Geometry: see drawing. Coordinates: mm, zero at the bounding-box minimum. A direction names the side the tool comes from. Coordinates: 2 decimals unless noted, no trailing zeros. One line per item, written item: value. Start each with the question number.
Item 1: Mould query, pull axis Z, two halves, no side actions, for the marked faces 4, 5, 6 and 7. Classes: released by +Z, released by -Z, zero draft, split by the parting line, or undercut.
Item 2: Pin query (flat end, axial travel): P1, Ø5, axis at x = 30.16, z = 4.76, coming from the -Y side; P2, Ø3, axis at y = 2, z = 3, coming from the -X side; P3, Ø3, axis at x = 31, y = 2, coming from the +Z side (1 decimal); P4, Ø3, axis at y = 1.5, z = 26.5, coming from the +X side (1 decimal). Return the tip coordinate at first contact, or that it passes through.
Item 3: Set-up query: the marked faces 1, 2 and 3. Return all of +Z, -Z, +X, -X, +Y, -Y with unobstructed straight access to the full face (end or side cutting, diameter ignored); none if empty.
Item 4: Ray query, L1, parallel to X at y = 2.5, z = 23 (1 decimal); L2, parallel to Z at x = 17.5, y = 5.75 (1 decimal); L3, parallel to Z at x = 7.5, y = 4.75 (1 decimal). Return the intervals inside material, ascending. Write a range as from..to.
Item 5: Cut plane B-B, the plane y = 2. State how many separate pieces and enclosed holes the cut face has, then the cut area to 3 significant figures.
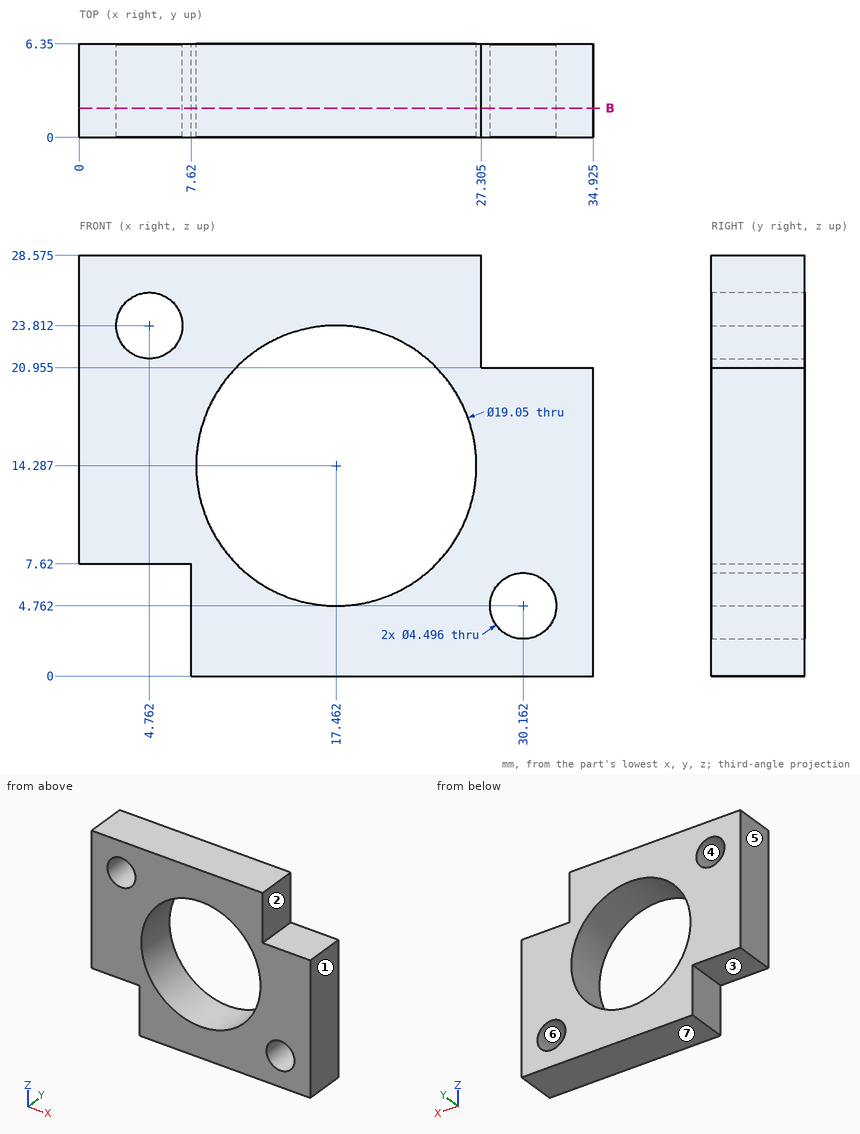
From the geometry:
1. face 4: undercut
1. face 5: zero draft
1. face 6: undercut
1. face 7: released by -Z
2. P1: stops at y = 0
2. P2: stops at x = 7.62
2. P3: stops at z = 21
2. P4: stops at x = 27.3
3. face 1: +Z, -Z, +X, +Y, -Y
3. face 2: +Z, +X, +Y, -Y
3. face 3: -Z, -X, +Y, -Y
4. L1: x = 0..2.7, 6.9..13.6, 21.3..27.3
4. L2: z = 0..4.8, 23.8..28.6
4. L3: z = 7.6..28.6
5. separate pieces: 1
5. enclosed holes: 3
5. area: 565 mm²
